Source: CAD feature listing. Evaluate the final solid. Frame: model axes, mm. A direction names the side the tool comes from. Coordinates: 2 decimals unless noted, no trailing zeros. Order: outer loops, then holes, each group sorted by start corner. A loop starts at its lowest first (then second) coordinate and runs counter-clockwise, first axis right, second up.
```python
from build123d import *

# Parameters (mm, degrees)
AUFSATZ_LINEAR_AUSTRAGEN1_DEPTH      = 461
AUFSATZ_LINEAR_AUSTRAGEN1_DEPTH_BACK = 60
SCHNITT_LINEAR_AUSTRAGEN1_DEPTH      = 468.275079584
SCHNITT_LINEAR_AUSTRAGEN1_DEPTH_BACK = 468.275079584
SKIZZE3_R                            = 27
LINEARES_MUSTER2_COUNT               = 2
LINEARES_MUSTER2_PITCH               = 60
LINEARES_MUSTER2_COUNT_DIR2          = 2
LINEARES_MUSTER2_PITCH_DIR2          = 30


with BuildPart() as part:
    # Skizze1 → Aufsatz-Linear austragen1 (new, two sides: drawn at the far end of the back side and taken through both)
    with BuildSketch(Plane(origin=(0, 0, 0), x_dir=(1, 0, 0), z_dir=(0, 1, 0)).offset(-AUFSATZ_LINEAR_AUSTRAGEN1_DEPTH_BACK)):
        with BuildLine():
            Line((-27.4, -65), (27.4, -65))
            ThreePointArc((27.4, -65), (36.309545443, -61.309545443), (40, -52.4))
            Line((40, -52.4), (40, 52.4))
            ThreePointArc((40, 52.4), (36.309545443, 61.309545443), (27.4, 65))
            Line((27.4, 65), (-27.4, 65))
            ThreePointArc((-27.4, 65), (-36.309545443, 61.309545443), (-40, 52.4))
            Line((-40, 52.4), (-40, -52.4))
            ThreePointArc((-40, -52.4), (-36.309545443, -61.309545443), (-27.4, -65))
        make_face()
        with BuildLine():
            Line((-27.4, -58.7), (27.4, -58.7))
            ThreePointArc((27.4, -58.7), (31.854772721, -56.854772721), (33.7, -52.4))
            Line((33.7, -52.4), (33.7, 52.4))
            ThreePointArc((33.7, 52.4), (31.854772721, 56.854772721), (27.4, 58.7))
            Line((27.4, 58.7), (-27.4, 58.7))
            ThreePointArc((-27.4, 58.7), (-31.854772721, 56.854772721), (-33.7, 52.4))
            Line((-33.7, 52.4), (-33.7, -52.4))
            ThreePointArc((-33.7, -52.4), (-31.854772721, -56.854772721), (-27.4, -58.7))
        make_face(mode=Mode.SUBTRACT)
    extrude(amount=AUFSATZ_LINEAR_AUSTRAGEN1_DEPTH + AUFSATZ_LINEAR_AUSTRAGEN1_DEPTH_BACK)

    # Skizze3 → Schnitt-Linear austragen1 (cut, two sides: drawn at the far end of the back side and taken through both)
    with BuildSketch(Plane.XY.offset(-SCHNITT_LINEAR_AUSTRAGEN1_DEPTH_BACK)):
        Circle(SKIZZE3_R)
    extrude(amount=SCHNITT_LINEAR_AUSTRAGEN1_DEPTH + SCHNITT_LINEAR_AUSTRAGEN1_DEPTH_BACK, mode=Mode.SUBTRACT)

    # Skizze7 → M10 Gewindebohrung2 (revolve, cut)
    with BuildSketch(Plane(origin=(40, -15, 30), x_dir=(0, 0, -1), z_dir=(0, 1, 0))):
        Polygon((0, 0), (0, 30.053657631), (4.25, 27.5), (4.25, 0), align=None)
    m10_gewindebohrung2 = revolve(axis=Axis((46.35, -15, 30), (-1, 0, 0)), mode=Mode.SUBTRACT)

    # Lineares Muster2: M10 Gewindebohrung2 2 × 2
    with Locations(*[(0, j * LINEARES_MUSTER2_PITCH_DIR2, -i * LINEARES_MUSTER2_PITCH) for i in range(LINEARES_MUSTER2_COUNT) for j in range(LINEARES_MUSTER2_COUNT_DIR2) if (i, j) != (0, 0)]):
        add(m10_gewindebohrung2, mode=Mode.SUBTRACT)


solid = part.part
```
1. Draft query along X for faces 1 (the face through (-36.21, 196.85, -61.41)), 2 (the face through (36.21, 196.85, 61.41)), 3 (the face through (0, 197, -58.7)). Return one class per face: released by +X, released by -X, zero draft, split by the parting line, or undercut.
Findings:
face 1: released by -X
face 2: released by +X
face 3: undercut
2. Pin query (flat end, axial travel): P1, Ø11, axis at y = -15, z = -30, coming from the +X side. Return the tip coordinate at first contact, or that it passes through.
Findings:
P1: stops at x = 40
3. Ray query, line 1 (X direction, y = 325, z = 38.5); line 2 (Z direction, x = 0.5, y = 221.5); line 3 (Z direction, x = 38, y = -15). Return the intervals inside material, ascending.
Findings:
line 1: x = -40 to -33.7, 33.7 to 40
line 2: z = -65 to -58.7, 58.7 to 65
line 3: z = -59.21 to -34.25, -25.75 to 25.75, 34.25 to 59.21
4. Section query B-B on y = 350.5. Return loops of the section in (x, z).
Findings:
outline: (-40, -52.4) arc R12.6 ccw to (-27.4, -65) - (27.4, -65) arc R12.6 ccw to (40, -52.4) - (40, 52.4) arc R12.6 ccw to (27.4, 65) - (-27.4, 65) arc R12.6 ccw to (-40, 52.4) - close; hole (-33.7, -52.4) arc R6.3 ccw to (-27.4, -58.7) - (27.4, -58.7) arc R6.3 ccw to (33.7, -52.4) - (33.7, 52.4) arc R6.3 ccw to (27.4, 58.7) - (-27.4, 58.7) arc R6.3 ccw to (-33.7, 52.4) - close
5. Section query C-C on z = 15. Return loops of the section in (x, y).
Findings:
outline: (-40, -60) - (-33.7, -60) - (-33.7, 461) - (-40, 461) - close; (33.7, -60) - (40, -60) - (40, 461) - (33.7, 461) - close
6. Access query for faces 4 (the face through (36.89, 17.59, 33.37)), 5 (the face through (-5.85, -26.36, 61.81)), 6 (the face through (-33.7, 197, -1)). Directions: +Z, -Z, +X, -X, +Y, -Y. A direction counts if a zero-diameter tool reaches every point of the face in a straight line with its end or side. Return the directions, or none.
Findings:
face 4: +X
face 5: +Z, -Z
face 6: +Y, -Y
7. Section query A-A on x = 0. Return loops of the section in (y, z), plus the area to 3 significant figures.
Findings:
outline: (-60, -65) - (-27, -65) - (-27, -58.7) - (-60, -58.7) - close; (-60, 58.7) - (-27, 58.7) - (-27, 65) - (-60, 65) - close; (27, -65) - (461, -65) - (461, -58.7) - (27, -58.7) - close; (27, 58.7) - (461, 58.7) - (461, 65) - (27, 65) - close
area: 5,880 mm2
8. Section query D-D on x = 20. Return loops of the section in (y, z).
Findings:
outline: (-60, -65) - (-18.14, -65) - (-18.14, -58.7) - (-60, -58.7) - close; (-60, 58.7) - (-18.14, 58.7) - (-18.14, 65) - (-60, 65) - close; (18.14, -65) - (461, -65) - (461, -58.7) - (18.14, -58.7) - close; (18.14, 58.7) - (461, 58.7) - (461, 65) - (18.14, 65) - close
